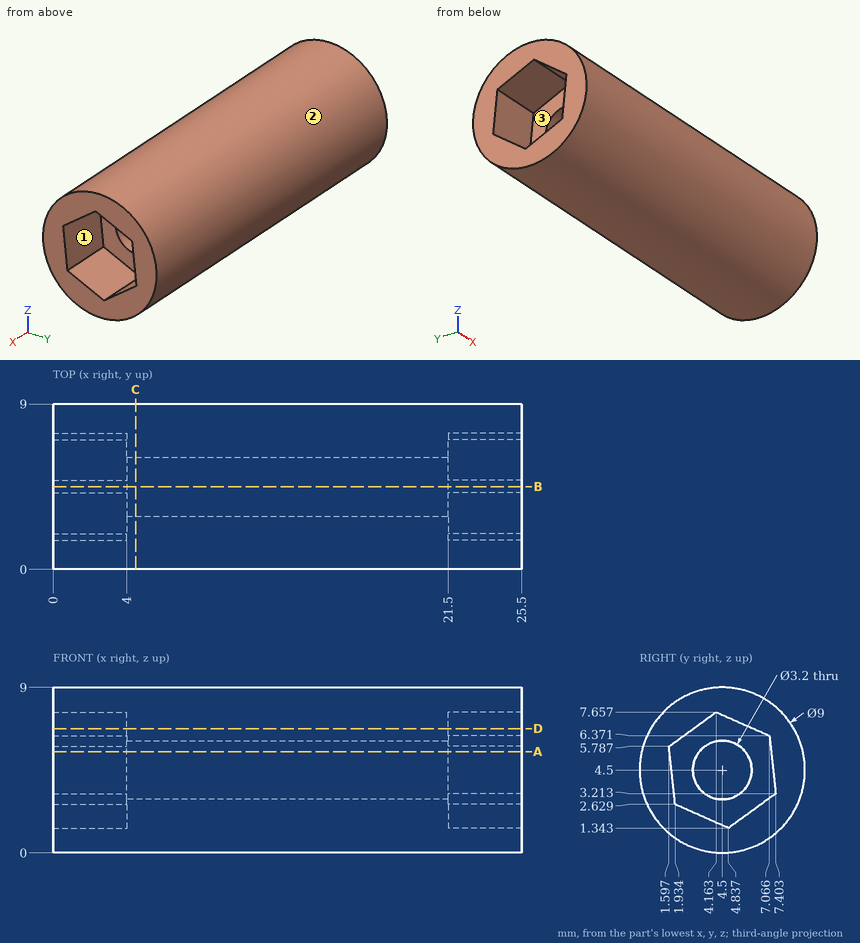
Print and shaded views of the part. All mm, measured from the part's lowest x, y and z. A direction names the side the tool comes from. Round coordinates to 2 decimals unless told otherwise and drop trailing zeros. Loops run counter-clockwise (first coordinate to the right, second up) from the corner with the lowest first, then second, coordinate; pieces in that order, holes last. Notation, with made-up numbers: (31.5, -35) -> (60.5, -35) arc R10 cw to (60.5, -17) -> close; hole circle Ø4 at (19, -30.75). An arc over 180 degrees is marked (long way). Use CSV: the item, a comma, the result in double quotes. Start each with the question number.
1) Cut at B-B, the plane y = 4.5. Write the cut outline in (x, z).
2) Cut at C-C, the plane x = 4.5. Write the cut outline in (y, z).
3) Cut at D-D, the plane z = 6.75. Write the cut outline in (x, y).
4) Which spindle directions (+Z, -Z, +X, -X, +Y, -Y) get a long thin tool onto all of the face, cutting with end or side? Do the marked faces 1, 2 and 3. Say none if no direction does.
5) Drop flat-ended pins along their axis: P1, Ø2.5, axis at y = 4.5, z = 4.5, coming from the +X side; P2, Ø5, axis at x = 9.5, z = 1, coming from the +Y side; P3, Ø1, axis at x = 4, y = 7.5, coming from the -Z side. Give the stop position or say it passes through.
6) Wall check: L1, parallel to Y at x = 10, z = 4.5; L2, parallel to Y at x = 12, z = 3.25 (1 decimal); L3, parallel to Z at x = 20, y = 5. Give the ranges that are in metal, low to high. Write a range as [from, to].
7) Cut at A-A, the plane z = 5.5. Write the cut outline in (x, y), plus the area to 3 significant figures.
Determined:
1,outline,"(0, 0) -> (25.5, 0) -> (25.5, 1.49) -> (21.5, 1.49) -> (21.5, 2.9) -> (4, 2.9) -> (4, 1.49) -> (0, 1.49) -> close; (0, 7.51) -> (4, 7.51) -> (4, 6.1) -> (21.5, 6.1) -> (21.5, 7.51) -> (25.5, 7.51) -> (25.5, 9) -> (0, 9) -> close"
2,outline,"circle Ø9 at (4.5, 4.5); hole circle Ø3.2 at (4.5, 4.5)"
3,outline,"(0, 0.6) -> (25.5, 0.6) -> (25.5, 2.92) -> (21.5, 2.92) -> (21.5, 6.21) -> (25.5, 6.21) -> (25.5, 8.4) -> (0, 8.4) -> (0, 6.21) -> (4, 6.21) -> (4, 2.92) -> (0, 2.92) -> close"
4,face 1,"+X"
4,face 2,"+X, -X"
4,face 3,"-X"
5,P1,"passes through"
5,P2,"stops at y = 8.89"
5,P3,"stops at z = 0.76"
6,L1,"y = [0, 2.9], [6.1, 9]"
6,L2,"y = [0.2, 3.5], [5.5, 8.8]"
6,L3,"z = [0.03, 2.98], [6.02, 8.97]"
7,outline,"(0, 0.11) -> (25.5, 0.11) -> (25.5, 1.63) -> (21.5, 1.63) -> (21.5, 3.25) -> (4, 3.25) -> (4, 1.63) -> (0, 1.63) -> close; (0, 7.16) -> (4, 7.16) -> (4, 5.75) -> (21.5, 5.75) -> (21.5, 7.16) -> (25.5, 7.16) -> (25.5, 8.89) -> (0, 8.89) -> close"
7,area,"136 mm2"
